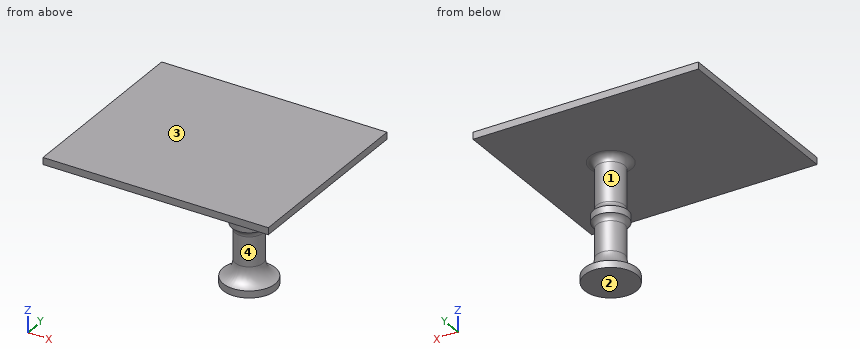
from build123d import *

# Parameters (mm, degrees)
SKIZZE2_W                       = 65
SKIZZE2_H                       = 100
AUFSATZ_LINEAR_AUSTRAGEN1_DEPTH = 2
SKIZZE3_R                       = 4
AUFSATZ_LINEAR_AUSTRAGEN2_DEPTH = 15
SKIZZE4_R                       = 5
AUFSATZ_LINEAR_AUSTRAGEN3_DEPTH = 2
SKIZZE5_R                       = 4
AUFSATZ_LINEAR_AUSTRAGEN4_DEPTH = 15
SKIZZE6_R                       = 7.5
AUFSATZ_LINEAR_AUSTRAGEN5_DEPTH = 2
VERRUNDUNG1_R                   = 2
VERRUNDUNG2_R                   = 2
VERRUNDUNG3_R                   = 5
SKIZZE7_W                       = 65
SKIZZE7_H                       = 45
SCHNITT_LINEAR_AUSTRAGEN1_DEPTH = 2
VERRUNDUNG4_R                   = 2


with BuildPart() as part:
    # Skizze2 → Aufsatz-Linear austragen1 (new body)
    with BuildSketch(Plane.XY):
        Rectangle(SKIZZE2_W, SKIZZE2_H)
    extrude(amount=AUFSATZ_LINEAR_AUSTRAGEN1_DEPTH)

    # Skizze3 → Aufsatz-Linear austragen2 (add)
    with BuildSketch(Plane(origin=(9.884440789, -5.646814133, 0), x_dir=(-1, 0, 0), z_dir=(0, 0, -1))):
        with Locations(Location((0, 28.149559508, 0), (0, 0, 180))):
            Circle(SKIZZE3_R)
    extrude(amount=AUFSATZ_LINEAR_AUSTRAGEN2_DEPTH)

    # Skizze4 → Aufsatz-Linear austragen3 (add)
    with BuildSketch(Plane(origin=(9.884440789, -5.646814133, -15), x_dir=(-1, 0, 0), z_dir=(0, 0, -1))):
        with Locations((0, 28.149559508)):
            Circle(SKIZZE4_R)
    extrude(amount=AUFSATZ_LINEAR_AUSTRAGEN3_DEPTH)

    # Skizze5 → Aufsatz-Linear austragen4 (add)
    with BuildSketch(Plane(origin=(9.884440789, -5.646814133, -17), x_dir=(-1, 0, 0), z_dir=(0, 0, -1))):
        with Locations(Location((0, 28.149559508, 0), (0, 0, 180))):
            Circle(SKIZZE5_R)
    extrude(amount=AUFSATZ_LINEAR_AUSTRAGEN4_DEPTH)

    # Skizze6 → Aufsatz-Linear austragen5 (add)
    with BuildSketch(Plane(origin=(9.884440789, -5.646814133, -32), x_dir=(-1, 0, 0), z_dir=(0, 0, -1))):
        with Locations((0, 28.149559508)):
            Circle(SKIZZE6_R)
    extrude(amount=AUFSATZ_LINEAR_AUSTRAGEN5_DEPTH)

    # Verrundung1
    # the kernel refuses this fillet: 2 mm, written as the material it adds along each edge
    with BuildSketch(Plane(origin=(9.884440789, 22.502745375, -15), x_dir=(1, 0, 0), z_dir=(0, 1, 0))) as verrundung1_piece_1:
        with BuildLine():
            CenterArc((6, -1.732050808), VERRUNDUNG1_R, 120, 60)
            Line((4, -1.732050808), (3.96, -1.732050808))
            Line((3.96, -1.732050808), (3.96, 0))
            Line((3.96, 0), (4, 0.04))
            ThreePointArc((4, 0.04), (4.5, 0.04), (4.98, 0.034641016))
            Line((4.98, 0.034641016), (5, 0))
        make_face()
    revolve(axis=Axis((9.884440789, 22.502745375, -15), (0, 0, -1)))

    # Verrundung2
    # the kernel refuses this fillet: 2 mm, written as the material it adds along each edge
    with BuildSketch(Plane(origin=(9.884440789, 22.502745375, -17), x_dir=(1, 0, 0), z_dir=(0, 1, 0))) as verrundung2_piece_1:
        with BuildLine():
            CenterArc((6, 1.732050808), VERRUNDUNG2_R, 180, 60)
            Line((4, 1.732050808), (3.96, 1.732050808))
            Line((3.96, 1.732050808), (3.96, 0))
            Line((3.96, 0), (4, -0.04))
            ThreePointArc((4, -0.04), (4.5, -0.04), (4.98, -0.034641016))
            Line((4.98, -0.034641016), (5, 0))
        make_face()
    revolve(axis=Axis((9.884440789, 22.502745375, -17), (0, 0, -1)))

    # Verrundung3
    # the kernel refuses this fillet: 5 mm, written as the material it adds along each edge
    with BuildSketch(Plane(origin=(9.884440789, 22.502745375, -32), x_dir=(1, 0, 0), z_dir=(0, 1, 0))) as verrundung3_piece_1:
        with BuildLine():
            CenterArc((9, -4.769696007), VERRUNDUNG3_R, 107.457603124, 72.542396876)
            Line((7.5, 0), (7.47, 0.09539392))
            ThreePointArc((7.47, 0.09539392), (5.75, 0.1), (4, 0.1))
            Line((4, 0.1), (3.9, 0))
            Line((3.9, 0), (3.9, -4.769696007))
            Line((3.9, -4.769696007), (4, -4.769696007))
        make_face()
    revolve(axis=Axis((9.884440789, 22.502745375, -32), (0, 0, -1)))

    # Skizze7 → Schnitt-Linear austragen1 (cut)
    with BuildSketch(Plane(origin=(0, 0, 0), x_dir=(-1, 0, 0), z_dir=(0, 0, -1))):
        with Locations((0, -27.5)):
            Rectangle(SKIZZE7_W, SKIZZE7_H)
    extrude(amount=-SCHNITT_LINEAR_AUSTRAGEN1_DEPTH, mode=Mode.SUBTRACT)

    # Verrundung4
    verrundung4_edges = [part.edges().sort_by_distance(p)[0] for p in [
        (5.884440789, 22.502745375, 0),
    ]]
    fillet(verrundung4_edges, radius=VERRUNDUNG4_R)


solid = part.part
The listing builds one solid part. Answer for the finished solid, in the listing's coordinates (mm). Face numbers are marked on the shaded views. Give positions to 0.01 mm unless a question says otherwise; leave off trailing zeros. Loops run counter-clockwise (first coordinate to the right, second up) from the corner with the lowest first, then second, coordinate; pieces in that order, holes last. Notation, with made-up numbers: (81.25, -14) - (89.25, -14) arc R22 cw to (89.25, -7) - close; hole circle Ø5 at (84, -10). An arc over 180 degrees is marked (long way). Use one line per item in the form item = value.
1. Given pin 1 Ø12 at (y, z) = (23.5, -21.5) entering from +X; pin 2 Ø1 at (x, y) = (10.5, 14) entering from -Z; pin 3 Ø1.5 at (x, z) = (16, -12) entering from +Y, each flat-ended and moving along its own axis, determine where each tip first touches the part or whether it passes through.
Calculated:
pin_1 = 14.88
pin_2 = 0
pin_3 = through
2. Section C-C on z = -11 is taken. Give the vertices of the cut face in (x, y).
Calculated:
outline = circle Ø8 at (9.88, 22.5)
3. Section A-A on x = -15 is taken. Give the vertices of the cut face in (y, z), then the cut area to 3 significant figures.
Calculated:
outline = (-5, 0) - (50, 0) - (50, 2) - (-5, 2) - close
area = 110 mm^2
4. Find the intervals of material crossed by line 1 along Z through (x, y) = (2.5, 10.5); line 2 along X through (y, z) = (23, -8.5); line 3 along X through (y, z) = (24, -4.5), in increasing order. Write a range as [from, to].
Calculated:
line_1 = [0, 2]
line_2 = [5.92, 13.85]
line_3 = [6.18, 13.59]
5. Section B-B on y = 36 is taken. Give the vertices of the cut face in (x, z).
Calculated:
outline = (-32.5, 0) - (32.5, 0) - (32.5, 2) - (-32.5, 2) - close
6. The mould has two halves that part along Z. Classify the marked faces 1, 2, 3 and 4: pulls with the +Z half, pulls with the -Z half, needs draft (parallel to the pull), parting line crosses it, or undercut.
Calculated:
face_1 = undercut
face_2 = pulls with the -Z half
face_3 = pulls with the +Z half
face_4 = undercut
